Check sheet for the modelled part. Datum: model origin and axes. Units: mm. Round coordinates to 2 decimals unless told otherwise and drop trailing zeros. Write each loop counter-clockwise with the first axis right and the second up, starting at its lowest first coordinate (ties: lowest second). Pieces come first, ordered by that corner, then holes.
Item 1: Cross-section at B-B on y = -53.5. Enter the section's corners in (x, z).
Item 2: Cross-section at A-A on y = -526.5. Enter the section's corners in (x, z), plus the area to 3 significant figures.
Item 3: Go/stop test with flat-tipped pins: pin 1 Ø2 at (y, z) = (-211, -1.5) entering from -X (3 decimals); pin 2 Ø2 at (y, z) = (-556, 21.5) entering from +X; pin 3 Ø3 at (y, z) = (-431, 17.5) entering from +X. Record where each tip stops, or that it passes through.
Item 4: Material ranges on line 1 (Y direction, x = -8.5, z = 18.5); line 2 (Z direction, x = 2, y = -368); line 3 (Z direction, x = 1.5, y = -476), recorded low to high.
from build123d import *

# Parameters (mm, degrees)
F1_DEPTH = 600
F3_DEPTH = 150
F4_R     = 4.99999


# Not quite as in the source:
# - a fillet or chamfer is up to 0.001 mm smaller than in the source, because OpenCascade refuses the exact size


with BuildPart() as f1:
    # F0 (on Front) → F1 (new body)
    with BuildSketch(Plane.XZ):
        with BuildLine():
            ThreePointArc((-5, 24.4948974278), (-15.8113883008, -19.364916731), (25, 0))
            ThreePointArc((25, 0), (19.364916731, 15.8113883008), (5, 24.4948974278))
            Line((5, 24.4948974278), (5, 20))
            Line((5, 20), (0, 20))
            Line((0, 20), (-5, 20))
            Line((-5, 20), (-5, 24.4948974278))
        make_face()
        with BuildLine():
            Line((5, 20), (5, 24.4948974278))
            ThreePointArc((5, 24.4948974278), (0, 25), (-5, 24.4948974278))
            Line((-5, 24.4948974278), (-5, 20))
            Line((-5, 20), (0, 20))
            Line((0, 20), (5, 20))
        make_face()
    extrude(amount=F1_DEPTH)

    # F2 (on face) → F3 (cut)
    with BuildSketch(Plane.XZ.offset(600)):
        with BuildLine():
            Line((-5, 20), (0, 20))
            Line((0, 20), (5, 20))
            Line((5, 20), (5, 24.4948974278))
            ThreePointArc((5, 24.4948974278), (0, 25), (-5, 24.4948974278))
            Line((-5, 24.4948974278), (-5, 20))
        make_face()
    extrude(amount=-F3_DEPTH, mode=Mode.SUBTRACT)

    # F4 (radius 5 in the source; OpenCascade refuses exactly that, so slightly less here)
    f4_edges = [f1.edges().sort_by_distance(p)[0] for p in [
        (-15.811388, -600, -19.364917),
    ]]
    fillet(f4_edges, radius=F4_R)


solid = f1.part
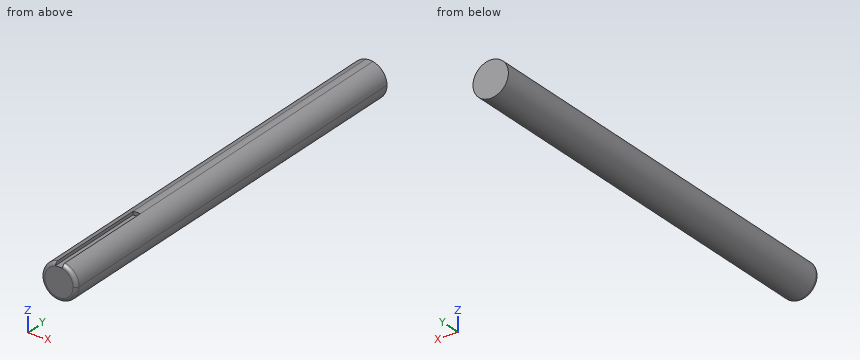
Response values:
1. outline: circle Ø50 at (0, 0)
2. outline: (-5, 20) - (-5, 24.49) arc R25 ccw (long way) to (5, 24.49) - (5, 20) - close
2. area: 1,920 mm2
3. pin 1: stops at x = -24.995
3. pin 2: stops at x = 14.31
3. pin 3: stops at x = 19.21
4. line 1: y = -599.99 to 0
4. line 2: z = -24.92 to 24.92
4. line 3: z = -24.95 to 20
